The model under review builds one solid part; all positions refer to its coordinate system, in mm. A direction names the side the tool comes from. Give positions to 0.01 mm unless a question says otherwise; leave off trailing zeros. Order: outer loops, then holes, each group sorted by start corner. A loop starts at its lowest first (then second) coordinate and runs counter-clockwise, first axis right, second up. Notation, with made-up numbers: (-31, 16.5) - (-20, 16.5) arc R11 cw to (-20, 37.5) - close; hole circle Ø1 at (-33, 0). An arc over 180 degrees is marked (long way). Write item = value, one per line. Start each with the question number.
1. We need section D-D, the plane y = -32. Give the boundary of the cut face in (x, z).
2. We need section A-A, the plane x = -1.5. Give the boundary of the cut face in (y, z), and give its area (3 significant figures).
3. We need section C-C, the plane z = 12.5. Give the boundary of the cut face in (x, y).
4. Machinability: for faces 4 (the flat face through (-25, -10.967, 13)), 5 (the flat face through (-22, -18.467, 13)), 6 (the flat face through (-21, -13, 23.8)), which of the approach directions +Z, -Z, +X, -X, +Y, -Y give a long, thin tool a straight path to every point of the face, cutting with its end or side? Answer none if there is none.
5. Wall thickness on probe 1 along Z at (x, y) = (-21.5, -18); probe 2 along Y at (x, z) = (0, 21.25); probe 3 along X at (y, z) = (-30, 18.75): over which ranges is each line inside the solid? List them lowest first.
6. For P1, Ø3, axis at y = -13.47, z = 5, coming from the +X side; P2, Ø4, axis at x = -28.5, z = 10.5, coming from the +Y side; P3, Ø6, axis at x = -24.5, z = 7.5, coming from the -Y side; P4, Ø2, axis at x = 6, z = 12, coming from the +Y side, all flat-tipped, find the tip position at first contact; note any pin that passes through.
7. Mouldability with a two-part tool opening along X and no side actions: class faces 1 (the cylindrical face through (-6.928, -13.24, 22.735)), 2 (the flat face through (-19.5, -13, 7)), 3 (the flat face through (6, 0, 13)) as pulls with the +X half, pulls with the -X half, needs draft (parallel to the pull), parting line crosses it, or undercut.
8. We need section B-B, the plane y = 30. Give the boundary of the cut face in (x, z), and give its area (3 significant figures).
from build123d import *

# Parameters (mm, degrees)
ESBO_O1_R                = 7.65
RESSALTO_EXTRUS_O1_DEPTH = 26
ESBO_O4_R                = 1.75
CORTE_EXTRUS_O1_DEPTH    = 67.790717918
ESBO_O5_W                = 3
ESBO_O5_H                = 5.6
CORTE_EXTRUS_O2_DEPTH    = 25


with BuildPart() as part:
    # Esboço1 → Ressalto-extrusão1 (new body)
    with BuildSketch(Plane.XY):
        with BuildLine():
            Line((-6, 18.467437405), (-6, -8.467437405))
            Line((-6, -8.467437405), (-31, -8.467437405))
            Line((-31, -8.467437405), (-31, -18.467437405))
            Line((-31, -18.467437405), (-16.77276441, -18.467437405))
            ThreePointArc((-16.77276441, -18.467437405), (-12.645234664, -20.645470326), (-12.113663185, -25.282038126))
            ThreePointArc((-12.113663185, -25.282038126), (4.577544662, -42.16741899), (6, -18.467437405))
            Line((6, -18.467437405), (6, 18.467437405))
            ThreePointArc((6, 18.467437405), (0, 43), (-6, 18.467437405))
        make_face()
        with Locations(Location((0, 30, 0), (0, 0, 180))):
            Circle(ESBO_O1_R, mode=Mode.SUBTRACT)
        with Locations(Location((0, -30, 0), (0, 0, 180))):
            Circle(ESBO_O1_R, mode=Mode.SUBTRACT)
    extrude(amount=RESSALTO_EXTRUS_O1_DEPTH)

    # Esboço3 → Corte-Revolução1 (revolve, cut)
    with BuildSketch(Plane.ZY.offset(31)):
        Polygon((13, -8.467437405), (21, -8.467437405), (21, -10.967437405), (18.5, -10.967437405), (18.5, -15.967437405), (21, -15.967437405), (21, -18.467437405), (13, -18.467437405), align=None)
    revolve(axis=Axis((-31, -8.467437405, 13), (0, -1, 0)), mode=Mode.SUBTRACT)

    # Esboço4 → Corte-extrusão1 (cut, through all)
    with BuildSketch(Plane.ZY.offset(31)):
        with Locations((5, -13.467437405)):
            Circle(ESBO_O4_R)
        with Locations(Location((21, -13.467437405, 0), (0, 0, 270))):
            Circle(ESBO_O4_R)
    extrude(amount=-CORTE_EXTRUS_O1_DEPTH, mode=Mode.SUBTRACT)

    # Esboço5 → Corte-extrusão2 (cut)
    with BuildSketch(Plane(origin=(0, -8.467437405, 0), x_dir=(1, 0, 0), z_dir=(0, 1, 0))):
        with Locations((-21, -5)):
            Rectangle(ESBO_O5_W, ESBO_O5_H)
        with Locations((-21, -21)):
            Rectangle(ESBO_O5_W, ESBO_O5_H)
    extrude(amount=-CORTE_EXTRUS_O2_DEPTH, mode=Mode.SUBTRACT)


solid = part.part
Model answer:
q1.outline = (-12.85, 0) - (-7.38, 0) - (-7.38, 26) - (-12.85, 26) - close; (7.38, 0) - (12.85, 0) - (12.85, 26) - (7.38, 26) - close
q2.outline = (-42.91, 0) - (-37.5, 0) - (-37.5, 26) - (-42.91, 26) - close; (-22.5, 0) - (22.5, 0) - (22.5, 26) - (-22.5, 26) - close; (37.5, 0) - (42.91, 0) - (42.91, 26) - (37.5, 26) - close; hole circle Ø3.5 at (-13.47, 5); hole circle Ø3.5 at (-13.47, 21)
q2.area = 1,430 mm2
q3.outline = (-25.52, -15.97) - (-23.02, -15.97) - (-23.02, -18.47) - (-16.77, -18.47) arc R5 cw to (-12.11, -25.28) arc R13 ccw (long way) to (6, -18.47) - (6, 18.47) arc R13 ccw (long way) to (-6, 18.47) - (-6, -8.47) - (-23.02, -8.47) - (-23.02, -10.97) - (-25.52, -10.97) - close; hole circle Ø15.3 at (0, -30); hole circle Ø15.3 at (0, 30)
q4.face_4 = -X, +Y
q4.face_5 = +Z, -Z, -X, -Y
q4.face_6 = +Y, -Y
q5.probe_1 = 0 to 2.2, 7.8 to 18.2, 23.8 to 26
q5.probe_2 = -43 to -37.65, -22.35 to -15.2, -11.74 to 22.35, 37.65 to 43
q5.probe_3 = -13 to -7.65, 7.65 to 13
q6.P1 = through
q6.P2 = -10.97
q6.P3 = -18.47
q6.P4 = 42
q7.face_1 = needs draft
q7.face_2 = undercut
q7.face_3 = pulls with the +X half
q8.outline = (-13, 0) - (-7.65, 0) - (-7.65, 26) - (-13, 26) - close; (7.65, 0) - (13, 0) - (13, 26) - (7.65, 26) - close
q8.area = 278 mm2
